Part model, mm, in its own coordinate system. Face numbers are marked on the shaded views. Round coordinates to 2 decimals unless told otherwise and drop trailing zeros. Loops run counter-clockwise (first coordinate to the right, second up) from the corner with the lowest first, then second, coordinate; pieces in that order, holes last. Notation, with made-up numbers: M 7,47.5 L 37,47.5 A18 cw 37,80.5 Z; hole C 64,-23.5 d9. An arc over 180 degrees is marked long. Answer as CSV lines item,"result". Start each with the question number.
Item 1: Mould opens along Y. For the marked faces 1, 2 and 3 say: pulls with the +Y half, pulls with the -Y half, needs draft (parallel to the pull), parting line crosses it, or undercut.
Item 2: Band-saw the part on A-A (x = 65.5). Give the cut face in (y, z), and give its area (3 significant figures).
Item 3: Drop flat-ended pins along their axis: pin 1 Ø2.5 at (x, z) = (-222.5, 24) entering from -Y; pin 2 Ø10 at (x, z) = (222.5, 26.39) entering from -Y; pin 3 Ø6 at (x, y) = (-133, -23.5) entering from +Z; pin 4 Ø12.5 at (x, z) = (77.5, 410.5) entering from -Y. Give the stop position or say it passes through.
Item 4: Band-saw the part on B-B (z = 383.5). Give the cut face in (x, y), and give its area (3 significant figures).
Item 5: Band-saw the part on C-C (y = -59.5). Give the cut face in (x, z).
Item 6: Wall check: line 1 (X direction, y = 114, z = 368); line 2 (Y direction, x = -151, z = 188); line 3 (Z direction, x = 220, y = 78). Give the ranges that are in metal, low to high.
Item 7: Band-saw the part on D-D (x = -113). Give the cut face in (y, z), and give its area (3 significant figures).
```python
from build123d import *

# Parameters (mm, degrees)
F0_W      = 600
F0_H      = 400
F1_DEPTH  = 25
F2_W      = 600
F2_H      = 400
F2_W_2    = 550
F2_H_2    = 350
F3_DEPTH  = 400
F5_DEPTH  = 600.001
F6_W      = 600
F6_H      = 200
F7_DEPTH  = 25
F8_R      = 75
F8_R_2    = 3.81
F9_DEPTH  = 25.4
F10_DEPTH = 25.4


with BuildPart() as f1:
    # F0 (on Top) → F1 (new body)
    with BuildSketch(Plane.XY):
        Rectangle(F0_W, F0_H)
    extrude(amount=F1_DEPTH)

    # F2 (on face) → F3 (join)
    with BuildSketch(Plane.XY.offset(25)):
        Rectangle(F2_W, F2_H)
        Rectangle(F2_W_2, F2_H_2, mode=Mode.SUBTRACT)
    extrude(amount=F3_DEPTH)

    # F4 (on face) → F5 (cut, through all)
    with BuildSketch(Plane(origin=(-300, 0, 0), x_dir=(0, -1, 0), z_dir=(-1, 0, 0))):
        Polygon((200, 225), (200, 425), (0, 425), align=None)
    extrude(amount=-F5_DEPTH, mode=Mode.SUBTRACT)

    # F6 (on face) → F7 (join)
    with BuildSketch(Plane.XY.offset(425)):
        with Locations((0, 100)):
            Rectangle(F6_W, F6_H)
    extrude(amount=-F7_DEPTH)

    # F8 (on face) → F9 (cut)
    with BuildSketch(Plane.XZ.offset(200)):
        with Locations((-180, 100)):
            Circle(F8_R)
        with Locations((180, 100)):
            Circle(F8_R)
        with Locations((-95, 100)):
            Circle(F8_R_2)
        with Locations((-137.5, 173.612159)):
            Circle(F8_R_2)
        with Locations((-222.5, 173.612159)):
            Circle(F8_R_2)
        with Locations((-265, 100)):
            Circle(F8_R_2)
        with Locations((-222.5, 26.387841)):
            Circle(F8_R_2)
        with Locations((-137.5, 26.387841)):
            Circle(F8_R_2)
        with Locations((95, 100)):
            Circle(F8_R_2)
        with Locations((137.5, 26.387841)):
            Circle(F8_R_2)
        with Locations((222.5, 26.387841)):
            Circle(F8_R_2)
        with Locations((265, 100)):
            Circle(F8_R_2)
        with Locations((222.5, 173.612159)):
            Circle(F8_R_2)
        with Locations((137.5, 173.612159)):
            Circle(F8_R_2)
    extrude(amount=-F9_DEPTH, mode=Mode.SUBTRACT)

    # F8 (on face) → F10 (cut)
    with BuildSketch(Plane.XZ.offset(200)):
        with Locations((-180, 100)):
            Circle(F8_R)
        with Locations((180, 100)):
            Circle(F8_R)
        with Locations((-95, 100)):
            Circle(F8_R_2)
        with Locations((-137.5, 173.612159)):
            Circle(F8_R_2)
        with Locations((-222.5, 173.612159)):
            Circle(F8_R_2)
        with Locations((-265, 100)):
            Circle(F8_R_2)
        with Locations((-222.5, 26.387841)):
            Circle(F8_R_2)
        with Locations((-137.5, 26.387841)):
            Circle(F8_R_2)
        with Locations((95, 100)):
            Circle(F8_R_2)
        with Locations((137.5, 26.387841)):
            Circle(F8_R_2)
        with Locations((222.5, 26.387841)):
            Circle(F8_R_2)
        with Locations((265, 100)):
            Circle(F8_R_2)
        with Locations((222.5, 173.612159)):
            Circle(F8_R_2)
        with Locations((137.5, 173.612159)):
            Circle(F8_R_2)
    extrude(amount=-F10_DEPTH, mode=Mode.SUBTRACT)


solid = f1.part
```
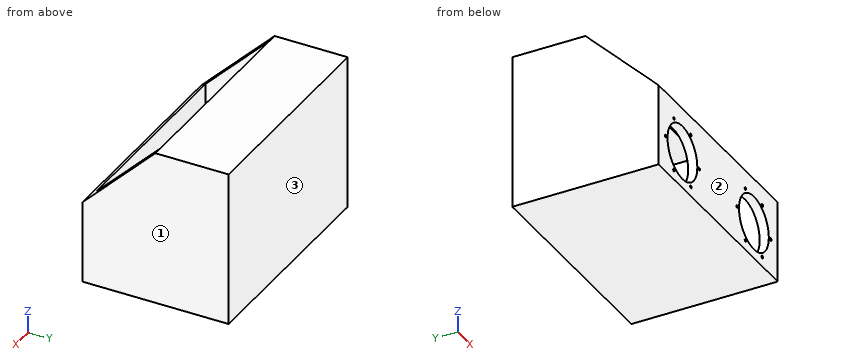
Answer block:
1,face 1,"needs draft"
1,face 2,"pulls with the -Y half"
1,face 3,"pulls with the +Y half"
2,outline,"M -200,0 L 200,0 L 200,425 L 0,425 L 0,400 L 175,400 L 175,25 L -175,25 L -175,250 L -200,225 Z"
2,area,"29,700 mm^2"
3,pin 1,"stops at y = -174.6"
3,pin 2,"stops at y = -200"
3,pin 3,"stops at z = 25"
3,pin 4,"stops at y = 0"
4,outline,"M -300,-41.5 L -275,-41.5 L -275,175 L 275,175 L 275,-41.5 L 300,-41.5 L 300,200 L -300,200 Z"
4,area,"25,800 mm^2"
5,outline,"M -300,0 L 300,0 L 300,365.5 L 275,365.5 L 275,25 L -275,25 L -275,365.5 L -300,365.5 Z"
6,line 1,"x = -300 to -275, 275 to 300"
6,line 2,"y = -200 to -175, 175 to 200"
6,line 3,"z = 0 to 25, 400 to 425"
7,outline,"M -200,0 L 200,0 L 200,425 L 0,425 L 0,400 L 175,400 L 175,25 L -175,25 L -175,66.3 L -200,66.3 Z; M -200,133.7 L -175,133.7 L -175,250 L -200,225 Z"
7,area,"28,000 mm^2"
